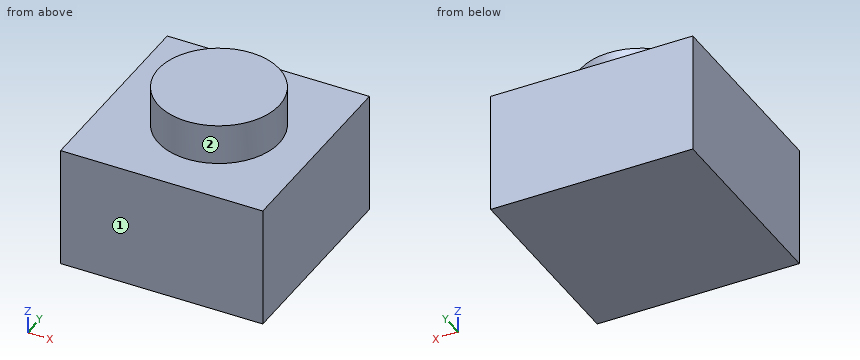
from build123d import *

# Parameters (mm, degrees)
F0_W     = 5
F0_H     = 5
F0_R     = 1.5
F1_DEPTH = 3
F2_DEPTH = 4


with BuildPart() as f1:
    # F0 (on Top) → F1 (new body)
    with BuildSketch(Plane.XY):
        with Locations((2.5, 35.520546)):
            Rectangle(F0_W, F0_H)
        with Locations((2.597283, 35.520546)):
            Circle(F0_R, mode=Mode.SUBTRACT)
        with Locations((2.597283, 35.520546)):
            Circle(F0_R)
    extrude(amount=F1_DEPTH)

    # F0 (on Top) → F2 (join)
    with BuildSketch(Plane.XY):
        with Locations((2.597283, 35.520546)):
            Circle(F0_R)
    extrude(amount=F2_DEPTH)


solid = f1.part
Here's how the part is built. I have some questions about the finished solid (model axes, mm). Face numbers are marked on the shaded views. A direction names the side the tool comes from. Round coordinates to 2 decimals unless told otherwise and drop trailing zeros. Order: outer loops, then holes, each group sorted by start corner. A loop starts at its lowest first (then second) coordinate and runs counter-clockwise, first axis right, second up. Notation, with made-up numbers: M 0,56 L 9,56 A14 cw 9,71 Z; hole C 75,76 d8. An arc over 180 degrees is marked long. One line per question, with ' | ' between items.
1) Imagine slicing it at C-C, the plane z = 3.65. Write out the boundary of the cut face in (x, y), plus the area to 3 significant figures.
Checked values:
outline: C 2.6,35.52 d3 | area: 7.07 mm²
2) Imagine slicing it at B-B, the plane y = 34.6. Write out the boundary of the cut face in (x, z), plus the area to 3 significant figures.
Checked values:
outline: M 0,0 L 5,0 L 5,3 L 3.78,3 L 3.78,4 L 1.41,4 L 1.41,3 L 0,3 Z | area: 17.4 mm²
3) Imagine slicing it at D-D, the plane y = 33.65. Write out the boundary of the cut face in (x, z).
Checked values:
outline: M 0,0 L 5,0 L 5,3 L 0,3 Z
4) Imagine slicing it at A-A, the plane x = 3.55. Write out the boundary of the cut face in (y, z), plus the area to 3 significant figures.
Checked values:
outline: M 33.02,0 L 38.02,0 L 38.02,3 L 36.68,3 L 36.68,4 L 34.36,4 L 34.36,3 L 33.02,3 Z | area: 17.3 mm²
5) On a 3-axis mill with a long thin cutter (end or side, diameter ignored), from which of +Z, -Z, +X, -X, +Y, -Y can I reach the whole of each face in a straight line? I mean the marked faces 1 and 2. Say none if no direction works.
Checked values:
face 1: +Z, -Z, +X, -X, -Y | face 2: +Z
6) I need wall thicknesses on line 1 (Z direction, x = 3.85, y = 34.25); line 2 (Y direction, x = 2, z = 3.1); line 3 (Y direction, x = 2.7, z = 3.3). Which ranges of each line are inside material? Lowest first, please.
Checked values:
line 1: z = 0 to 3 | line 2: y = 34.14 to 36.9 | line 3: y = 34.02 to 37.02
